Read the model definition and answer for the solid it produces. Units are mm, in the model's axes. A direction names the side the tool comes from. Round coordinates to 2 decimals unless told otherwise and drop trailing zeros. Loops run counter-clockwise (first coordinate to the right, second up) from the corner with the lowest first, then second, coordinate; pieces in that order, holes last. Notation, with made-up numbers: M -12.75,-17 L 20.25,-17 A19 ccw 20.25,-5 Z; hole C -12.75,68 d3. An arc over 180 degrees is marked long. Write each question's results on one line, items separated by ' | '.
```python
from build123d import *

# Parameters (mm, degrees)
SKICA2_W                = 12.5
SKICA2_H                = 9
P_IDAT_VYSUNUT_M1_DEPTH = 7.5
SKICA3_R                = 8.5
P_IDAT_VYSUNUT_M2_DEPTH = 6.5
SKICA4_W                = 0.8
SKICA4_H                = 4
P_IDAT_VYSUNUT_M3_DEPTH = 8


with BuildPart() as part:
    # Skica2 → Přidat vysunutím1 (new body)
    with BuildSketch(Plane(origin=(0, 0, 0), x_dir=(1, 0, 0), z_dir=(0, 1, 0))):
        Rectangle(SKICA2_W, SKICA2_H)
    extrude(amount=P_IDAT_VYSUNUT_M1_DEPTH)

    # Skica3 → Přidat vysunutím2 (add)
    with BuildSketch(Plane(origin=(0, 7.5, 0), x_dir=(1, 0, 0), z_dir=(0, 1, 0))):
        Circle(SKICA3_R)
    extrude(amount=P_IDAT_VYSUNUT_M2_DEPTH)

    # Skica4 → Přidat vysunutím3 (add)
    with BuildSketch(Plane(origin=(0, 0, 0), x_dir=(-1, 0, 0), z_dir=(0, -1, 0))):
        with Locations((5.3, 0)):
            Rectangle(SKICA4_W, SKICA4_H)
        Rectangle(SKICA4_W, SKICA4_H)
    extrude(amount=P_IDAT_VYSUNUT_M3_DEPTH)


solid = part.part
```
1. Which of the six approach directions +Z, -Z, +X, -X, +Y, -Y give full straight-line access (tool end or side, diameter ignored) to faces 5 (the face through (6.25, 4, 0)), 6 (the face through (-5.7, -4, 0)), 7 (the face through (-5.3, -3.9, 2)), 8 (the face through (0, 4, -4.5))?
Completed:
face 5: +Z, -Z, +X, -Y | face 6: +Z, -Z, -X, -Y | face 7: +Z, +X, -X, -Y | face 8: -Z, +X, -X, -Y
2. Find section C-C, the plane x = 0. Give the vertices of the cut face in (y, z), then the cut area to 3 significant figures.
Completed:
outline: M -8,-2 L 0,-2 L 0,-4.5 L 7.5,-4.5 L 7.5,-8.5 L 14,-8.5 L 14,8.5 L 7.5,8.5 L 7.5,4.5 L 0,4.5 L 0,2 L -8,2 Z | area: 210 mm2
3. Determine the mould class of faces 1 (the face through (-6.25, 4, 0)), 2 (the face through (-0.4, -4, 0)), 3 (the face through (0.4, -4, 0)), 4 (the face through (-4.9, -4, 0)) for opening direction X: released by +X, released by -X, zero draft, split by the parting line, or undercut.
Completed:
face 1: released by -X | face 2: undercut | face 3: released by +X | face 4: undercut
4. Find section A-A, the plane y = -5. Give the vertices of the cut face in (x, z), then the cut area to 3 significant figures.
Completed:
outline: M -5.7,-2 L -4.9,-2 L -4.9,2 L -5.7,2 Z; M -0.4,-2 L 0.4,-2 L 0.4,2 L -0.4,2 Z | area: 6.40 mm2
5. Given P1, Ø0.6, axis at x = 0, y = -4.5, coming from the +Z side; P2, Ø4, axis at x = 3, y = 4.5, coming from the -Z side; P3, Ø3, axis at y = -4.5, z = 0, coming from the -X side, each flat-ended and moving along its own axis, determine where each tip first touches the part or whether it passes through.
Completed:
P1: stops at z = 2 | P2: stops at z = -4.5 | P3: stops at x = -5.7
6. Find the intervals of material crossed by L1, parallel to X at y = -0.25, z = 1.25; L2, parallel to Y at x = -7.25, z = 4.25; L3, parallel to Y at x = 5.75, z = -3.5, in increasing order.
Completed:
L1: x = -5.7 to -4.9, -0.4 to 0.4 | L2: y = 7.5 to 14 | L3: y = 0 to 14
7. Find section D-D, the plane x = -4. Give the vertices of the cut face in (y, z), then the cut area to 3 significant figures.
Completed:
outline: M 0,-4.5 L 7.5,-4.5 L 7.5,-7.5 L 14,-7.5 L 14,7.5 L 7.5,7.5 L 7.5,4.5 L 0,4.5 Z | area: 165 mm2
8. Find section B-B, the plane z = 0. Give the vertices of the cut face in (x, y), then the cut area to 3 significant figures.
Completed:
outline: M -8.5,7.5 L -6.25,7.5 L -6.25,0 L -5.7,0 L -5.7,-8 L -4.9,-8 L -4.9,0 L -0.4,0 L -0.4,-8 L 0.4,-8 L 0.4,0 L 6.25,0 L 6.25,7.5 L 8.5,7.5 L 8.5,14 L -8.5,14 Z | area: 217 mm2
